The listing builds one solid part. Answer for the finished solid, in the listing's coordinates (mm). A direction names the side the tool comes from. Give positions to 0.01 mm unless a question says otherwise; leave off trailing zeros. Loops run counter-clockwise (first coordinate to the right, second up) from the corner with the lowest first, then second, coordinate; pieces in that order, holes last. Notation, with made-up numbers: (18.25, 64) - (69.25, 64) arc R18 ccw to (69.25, 74) - close; hole circle Ø5 at (-28, 83.5). An arc over 180 degrees is marked (long way). Answer as CSV lines item,"result". Start each with the question number.
1) A cutting plane is placed at B-B (z = 35.5). Give the number of separate pieces and of enclosed holes in the cut face, and give its area (3 significant figures).
2) Find the intervals of material crossed by line 1 along X through (y, z) = (43, 38.5); line 2 along Y through (x, z) = (-3.5, 7.5); line 3 along X through (y, z) = (25, 9), in increasing order.
3) For a pull along Y with two mould halves and no side action, classify faces 1 (the face through (-78, 54, 25)), 2 (the face through (-52.42, 14.64, 42.33)), 3 (the face through (-74, 59.6, 10)), 4 (the face through (74, 62, 25)) as pulls with the +Y half, pulls with the -Y half, needs draft (parallel to the pull), parting line crosses it, or undercut.
4) For faces 5 (the face through (-47.99, 14.43, 7.09)), 6 (the face through (76.3, 59.4, 40.3)), 7 (the face through (30.231, 8.794, 35.761)), 8 (the face through (74, 57, 25)), determine the directions among +Z, -Z, +X, -X, +Y, -Y from which every point of the face is accessible in a straight line to the end or side of a thin tool.
5) Flat-ended cylindrical pins translate along their axes: pin 1 (4.5 mm diameter, centred on x = 74, z = 27, fed in from -Y); pin 2 (12 mm diameter, centred on x = -12.5, z = 9.5, fed in from +Y); pin 3 (1.5 mm diameter, centred on x = 15, z = 25, fed in from +Y); pin 4 (16 mm diameter, centred on y = 59, z = 17, fed in from +X). Find the tip coordinate at first contact, or state that the pin passes through.
6) A cutting plane is placed at A-A (y = 59.5). Determine the outline of the cut face in (x, z), and give its area (3 significant figures).
```python
from build123d import *

# Parameters (mm, degrees)
BOSS_EXTRUDE1_DEPTH      = 50
FILLET1_R                = 10
FILLET2_R                = 18
CUT_EXTRUDE1_DEPTH       = 8
CHAMFER1_SIZE            = 2
CHAMFER2_SIZE            = 6
SKETCH3_R                = 17.75
CUT_EXTRUDE2_DEPTH       = 8
SKETCH4_R                = 20.25
CUT_EXTRUDE3_DEPTH       = 4
CHAMFER1_OF_MIRROR2_SIZE = 2
CHAMFER2_OF_MIRROR2_SIZE = 6


with BuildPart() as part:
    # Sketch1 → Boss-Extrude1 (new body)
    with BuildSketch(Plane.XY):
        Polygon((-15, 0), (15, 0), (70, 31.754264805), (70, 70), (78, 70), (78, 27.135462652), (17.143593539, -8), (-17.143593539, -8), (-78, 27.135462652), (-78, 70), (-70, 70), (-70, 31.754264805), align=None)
    extrude(amount=BOSS_EXTRUDE1_DEPTH)

    # Fillet1
    fillet1_edges = [part.edges().sort_by_distance(p)[0] for p in [
        (-15, 0, 25),
        (15, 0, 25),
        (70, 31.754264805, 25),
        (-70, 31.754264805, 25),
    ]]
    fillet(fillet1_edges, radius=FILLET1_R)

    # Fillet2
    fillet2_edges = [part.edges().sort_by_distance(p)[0] for p in [
        (78, 27.135462652, 25),
        (17.143593539, -8, 25),
        (-17.143593539, -8, 25),
        (-78, 27.135462652, 25),
    ]]
    fillet(fillet2_edges, radius=FILLET2_R)

    # Sketch2 → Cut-Extrude1 (cut)
    with BuildSketch(Plane(origin=(-78, 160.753072215, 0), x_dir=(0, 0, 1), z_dir=(1, 0, 0))):
        with BuildLine():
            Line((12.5, 103.753072215), (37.5, 103.753072215))
            ThreePointArc((37.5, 103.753072215), (40, 101.253072215), (37.5, 98.753072215))
            Line((37.5, 98.753072215), (12.5, 98.753072215))
            ThreePointArc((12.5, 98.753072215), (10, 101.253072215), (12.5, 103.753072215))
        make_face()
    cut_extrude1 = extrude(amount=CUT_EXTRUDE1_DEPTH, mode=Mode.SUBTRACT)

    # Chamfer1
    chamfer1_edges = [part.edges().sort_by_distance(p)[0] for p in [
        (-70, 59.5, 10),
        (-78, 59.5, 10),
        (-70, 62, 25),
        (-78, 62, 25),
        (-70, 59.5, 40),
        (-78, 59.5, 40),
        (-70, 57, 25),
        (-78, 57, 25),
    ]]
    chamfer(chamfer1_edges, length=CHAMFER1_SIZE)

    # Chamfer2
    chamfer2_edges = [part.edges().sort_by_distance(p)[0] for p in [
        (-74, 70, 50),
        (-74, 70, 0),
    ]]
    chamfer(chamfer2_edges, length=CHAMFER2_SIZE)

    # Sketch3 → Cut-Extrude2 (cut)
    with BuildSketch(Plane(origin=(-27.350055988, -2.107296158, 0), x_dir=(0, 0, 1), z_dir=(0.5, 0.866025404, 0))):
        with Locations(Location((25, -26.237677779, 0), (0, 0, 90))):  # turned: the seam where the file's is
            Circle(SKETCH3_R)
    cut_extrude2 = extrude(amount=CUT_EXTRUDE2_DEPTH, mode=Mode.SUBTRACT)

    # Sketch4 → Cut-Extrude3 (cut)
    with BuildSketch(Plane(origin=(-3.75, -6.495190528, 0), x_dir=(0, 0, -1), z_dir=(0.5, 0.866025404, 0))):
        with Locations(Location((-25, 48.869872981, 0), (0, 0, 90))):  # turned: the seam where the file's is
            Circle(SKETCH4_R)
    cut_extrude3 = extrude(amount=-CUT_EXTRUDE3_DEPTH, mode=Mode.SUBTRACT)

    # Mirror2: Cut-Extrude1, Cut-Extrude2, Cut-Extrude3 across plane
    add(cut_extrude1.mirror(Plane(origin=(0, 0, 0), x_dir=(0, 0, 1), z_dir=(1, 0, 0))), mode=Mode.SUBTRACT)
    add(cut_extrude2.mirror(Plane(origin=(0, 0, 0), x_dir=(0, 0, 1), z_dir=(1, 0, 0))), mode=Mode.SUBTRACT)
    add(cut_extrude3.mirror(Plane(origin=(0, 0, 0), x_dir=(0, 0, 1), z_dir=(1, 0, 0))), mode=Mode.SUBTRACT)

    # Chamfer1 of Mirror2
    chamfer1_of_mirror2_edges = [part.edges().sort_by_distance(p)[0] for p in [
        (70, 59.5, 10),
        (78, 59.5, 10),
        (70, 62, 25),
        (78, 62, 25),
        (70, 59.5, 40),
        (78, 59.5, 40),
        (70, 57, 25),
        (78, 57, 25),
    ]]
    chamfer(chamfer1_of_mirror2_edges, length=CHAMFER1_OF_MIRROR2_SIZE)

    # Chamfer2 of Mirror2
    chamfer2_of_mirror2_edges = [part.edges().sort_by_distance(p)[0] for p in [
        (74, 70, 50),
        (74, 70, 0),
    ]]
    chamfer(chamfer2_of_mirror2_edges, length=CHAMFER2_OF_MIRROR2_SIZE)


solid = part.part
```
Ans:
1,separate pieces,"5"
1,enclosed holes,"0"
1,area,"1,350 mm2"
2,line 1,"-78 to -70, 70 to 78"
2,line 2,"-8 to 0"
2,line 3,"-72.92 to -58.3, 58.3 to 72.92"
3,face 1,"needs draft"
3,face 2,"parting line crosses it"
3,face 3,"undercut"
3,face 4,"undercut"
4,face 5,"none"
4,face 6,"+X"
4,face 7,"+Z, -Z, +Y"
4,face 8,"+X, -X"
5,pin 1,"y = 23.89"
5,pin 2,"y = 2.02"
5,pin 3,"y = 0.61"
5,pin 4,"x = 78"
6,outline,"(-78, 0) - (-70, 0) - (-70, 8) - (-72, 10) - (-76, 10) - (-78, 8) - close; (-78, 42) - (-76, 40) - (-72, 40) - (-70, 42) - (-70, 50) - (-78, 50) - close; (70, 0) - (78, 0) - (78, 8) - (76, 10) - (72, 10) - (70, 8) - close; (70, 42) - (72, 40) - (76, 40) - (78, 42) - (78, 50) - (70, 50) - close"
6,area,"304 mm2"
